Geometry check sheet. Reference: the model listing, model coordinates, mm. A direction names the side the tool comes from. Round coordinates to 2 decimals unless told otherwise and drop trailing zeros. Order: outer loops, then holes, each group sorted by start corner. A loop starts at its lowest first (then second) coordinate and runs counter-clockwise, first axis right, second up.
```python
from build123d import *

# Parameters (mm, degrees)
SKETCH1_R            = 5
SKETCH1_R_2          = 4
BOSS_EXTRUDE1_DEPTH  = 3.5
BOSS_EXTRUDE2_DEPTH  = 3.5
M2_CLEARANCE_HOLE1_D = 2.6
SKETCH6_R            = 4
SKETCH6_R_2          = 3.25
BOSS_EXTRUDE4_DEPTH  = 1


with BuildPart() as part:
    # Sketch1 → Boss-Extrude1 (new body)
    with BuildSketch(Plane(origin=(0, 0, 0), x_dir=(1, 0, 0), z_dir=(0, 1, 0))):
        with Locations(Location((0, 0, 0), (0, 0, 270))):
            Circle(SKETCH1_R)
        with Locations(Location((0, 0, 0), (0, 0, 270))):
            Circle(SKETCH1_R_2, mode=Mode.SUBTRACT)
    extrude(amount=BOSS_EXTRUDE1_DEPTH)

    # Sketch2 → Boss-Extrude2 (add)
    with BuildSketch(Plane(origin=(0, 0, 0), x_dir=(1, 0, 0), z_dir=(0, 1, 0))):
        with BuildLine():
            Line((-7.892857143, 2.335124434), (-1.785714286, 4.670248868))
            ThreePointArc((-1.785714286, 4.670248868), (-5, 0), (-1.785714286, -4.670248868))
            Line((-1.785714286, -4.670248868), (-7.892857143, -2.335124434))
            ThreePointArc((-7.892857143, -2.335124434), (-9.5, 0), (-7.892857143, 2.335124434))
        make_face()
        with BuildLine():
            Line((7.892857143, -2.335124434), (1.785714286, -4.670248868))
            ThreePointArc((1.785714286, -4.670248868), (5, 0), (1.785714286, 4.670248868))
            Line((1.785714286, 4.670248868), (7.892857143, 2.335124434))
            ThreePointArc((7.892857143, 2.335124434), (9.5, 0), (7.892857143, -2.335124434))
        make_face()
    extrude(amount=BOSS_EXTRUDE2_DEPTH)

    # M2 Clearance Hole1 (through all)
    with Locations(Plane(origin=(0, 3.5, 0), x_dir=(1, 0, 0), z_dir=(0, 1, 0))):
        with Locations((-7, 0), (7, 0)):
            Hole(M2_CLEARANCE_HOLE1_D / 2)

    # Sketch6 → Boss-Extrude4 (add)
    with BuildSketch(Plane.XZ):
        with Locations(Location((0, 0, 0), (0, 0, 270))):
            Circle(SKETCH6_R)
        with Locations(Location((0, 0, 0), (0, 0, 270))):
            Circle(SKETCH6_R_2, mode=Mode.SUBTRACT)
    extrude(amount=-BOSS_EXTRUDE4_DEPTH)


solid = part.part
```
(1) Sectioned sample at D-D, the plane z = -3. Record the cut outline in (x, y), and give its area (3 significant figures).
Returned:
outline: (-6.15, 0) - (-1.25, 0) - (-1.25, 1) - (-2.65, 1) - (-2.65, 3.5) - (-6.15, 3.5) - close; (1.25, 0) - (6.15, 0) - (6.15, 3.5) - (2.65, 3.5) - (2.65, 1) - (1.25, 1) - close
area: 27.3 mm2
(2) Sectioned sample at A-A, the plane y = 2.7. Record the cut outline in (x, z).
Returned:
outline: (-7.89, -2.34) - (-1.79, -4.67) arc R5 ccw to (1.79, -4.67) - (7.89, -2.34) arc R2.5 ccw to (7.89, 2.34) - (1.79, 4.67) arc R5 ccw to (-1.79, 4.67) - (-7.89, 2.34) arc R2.5 ccw to start; hole circle Ø2.6 at (-7, 0); hole circle Ø8 at (0, 0); hole circle Ø2.6 at (7, 0)
(3) Draft check along X on faces 3 (the cylindrical face through (5.76, 1.73, -0.39)), 4 (the cylindrical face through (-8.24, 1.73, -0.39)), 5 (the flat face through (4.797, 1.726, -3.519)), 6 (the flat face through (-4.1, 3.5, 1)). Enter one of: released by +X, released by -X, zero draft, split by the parting line, or undercut.
Returned:
face 3: undercut
face 4: undercut
face 5: released by +X
face 6: zero draft
(4) Sectioned sample at C-C, the plane x = 0.5. Record the cut outline in (y, z).
Returned:
outline: (0, -4.97) - (3.5, -4.97) - (3.5, -3.97) - (1, -3.97) - (1, -3.21) - (0, -3.21) - close; (0, 3.21) - (1, 3.21) - (1, 3.97) - (3.5, 3.97) - (3.5, 4.97) - (0, 4.97) - close
(5) Depth check by flat-ended pin: P1, Ø1, axis at x = -2.5, y = 0.5, coming from the -Z side; P2, Ø2, axis at x = 6, y = 3, coming from the -Z side; P3, Ø2.5, axis at x = 7, z = 0, coming from the +Y side. Enter the tip coordinate at first touch or a pass-through.
Returned:
P1: stops at z = -4.59
P2: stops at z = -3.44
P3: passes through
(6) Sectioned sample at B-B, the plane z = 0. Record the cut outline in (x, y).
Returned:
outline: (-9.5, 0) - (-8.3, 0) - (-8.3, 3.5) - (-9.5, 3.5) - close; (-5.7, 0) - (-3.25, 0) - (-3.25, 1) - (-4, 1) - (-4, 3.5) - (-5.7, 3.5) - close; (3.25, 0) - (5.7, 0) - (5.7, 3.5) - (4, 3.5) - (4, 1) - (3.25, 1) - close; (8.3, 0) - (9.5, 0) - (9.5, 3.5) - (8.3, 3.5) - close
(7) Set-up check for faces 1 (the cylindrical face through (-3.905, 2.232, -0.867)), 2 (the cylindrical face through (9.5, 1.7, 0)): record each of +Z, -Z, +X, -X, +Y, -Y from which the full face is reachable in a straight line by a thin tool's end or side.
Returned:
face 1: +Y
face 2: +X, +Y, -Y
(8) Material ranges on line 1 (Z direction, x = 0.25, y = 3); line 2 (X direction, y = 2.45, z = -0.25); line 3 (Z direction, x = 2.75, y = 2.8), recorded low to high.
Returned:
line 1: z = -4.99 to -3.99, 3.99 to 4.99
line 2: x = -9.49 to -8.28, -5.72 to -3.99, 3.99 to 5.72, 8.28 to 9.49
line 3: z = -4.3 to -2.9, 2.9 to 4.3
